Check sheet for the modelled part. Datum: model origin and axes. Units: mm. A direction names the side the tool comes from. Round coordinates to 2 decimals unless told otherwise and drop trailing zeros. Write each loop counter-clockwise with the first axis right and the second up, starting at its lowest first coordinate (ties: lowest second). Pieces come first, ordered by that corner, then holes. Notation, with made-up numbers: M 82.5,51 L 88.5,51 A16 ccw 88.5,73 Z; hole C -11.75,-38 d4. An arc over 180 degrees is marked long. Put each result on its own line as item: value.
Autodesk Inventor part; units mm, degrees
ref_plane "Work Plane1" through (0, 0, 0) normal (0, 0, 1) x (1, 0, 0)
ref_plane "Work Plane3" through (-57, -102.111, 0) normal (0, 1, 0) x (1, 0, 0)
ref_plane "YZ Plane" through (0, 0, 0) normal (1, 0, 0) x (0, 1, 0)
ref_plane "Work Plane1" through (0, 0, 0) normal (0, 0, 1) x (1, 0, 0)
sketch "Sketch1" plane through (0, 0, 0) normal (0, 0, 1) x (1, 0, 0)
  line L0 (-60, -142.911) -> (-60, -152.111) construction
  line L1 (0, -152.111) -> (-60, -152.111) construction
  line L2 (0, -142.911) -> (0, -152.111) construction
  line L3 (-57, -81.311) -> (-9.2, -81.311)
  line L4 (-9.2, -81.311) -> (-9.2, -142.911)
  line L5 (-9.2, -142.911) -> (-57, -142.911)
  line L6 (-57, -142.911) -> (-57, -81.311)
  line L7 (-57, -112.111) -> (-9.2, -112.111) construction
  line L8 (-57, -102.111) -> (-50, -102.111)
  line L9 (-50, -102.111) -> (-50, -122.111)
  line L10 (-50, -122.111) -> (-57, -122.111)
  line L11 (-57, -122.111) -> (-57, -102.111)
  line L12 (0, -142.911) -> (-60, -142.911)
  point P0 (0, 0)
  dimension "d0" = 20
  dimension "d1" = 7
extrude "Extrusion1" add sketch "Sketch1" against normal blind 1 contours L3 L4 L5 L6 L10 L9 L8
ref_plane "Work Plane2" through (-57, -112.111, 0) normal (0, 1, 0) x (1, 0, 0)
sketch "Sketch2" plane through (-57, -112.111, 0) normal (0, 1, 0) x (1, 0, 0)
  line L0 (7, 0) -> (0, 0) construction
  line L1 (7, 0) -> (7, 1) construction
  line L2 (0, 1) -> (7, 1) construction
  line L3 (0, 0) -> (0, 1) construction
  line L4 (0.0721, -0.8167) -> (0.0721, 1.0988)
  line L5 (0.0721, 1.0988) -> (-0.9279, 1.3644)
  line L6 (-0.9279, 1.3644) -> (0.0477, 5.0375)
  arc A0 (1.8249, 5.3661) -> (0.0477, 5.0375) centre (1.0142, 4.7807) ccw
  line L7 (1.8249, 5.3661) -> (4.3785, 1.8293)
  arc A1 (4.3785, 1.8293) -> (6, 1) centre (6, 3) ccw
  line L8 (6, 1) -> (7, 1)
  line L9 (7, 1) -> (7, 0)
  line L10 (7, 0) -> (6, 0)
  arc A2 (3.5677, 1.2439) -> (6, 0) centre (6, 3) ccw
  line L11 (3.5677, 1.2439) -> (1.0644, 4.7112)
  arc A3 (1.0644, 4.7112) -> (0.9749, 4.6822) centre (1.0243, 4.6822) ccw
  line L12 (47.8, 0) -> (0, 0)
  line L13 (47.8, 1) -> (0, 1)
  line L14 (6, 0) -> (6, 1) construction
  line L15 (0.9749, -0.9502) -> (0.9749, 4.6822)
  line L16 (0.2208, -1.01) -> (0.7236, -1.1435)
  arc A4 (0.7236, -1.1435) -> (0.9749, -0.9502) centre (0.7749, -0.9502) ccw
  arc A5 (0.0721, -0.8167) -> (0.2208, -1.01) centre (0.2721, -0.8167) ccw
  point P0 (57, 0)
  point P1 (0.9749, -1.2103)
  point P2 (0.0721, -0.9705)
  dimension "d8" = 1
  dimension "d9" = 1
  dimension "d11" = 1
  dimension "d12" = 0.0494
  dimension "d22" = 1
  dimension "d23" = 2
  dimension "d32" = 2
  dimension "d34" = 2.5
  dimension "d36" = 0.2
  dimension "d37" = 0.9874
  dimension "d38" = 1
  dimension "d39" = 125.829
  dimension "d40" = 3.8003
extrude "Extrusion2" add sketch "Sketch2" along normal mid plane 16 contours L4 L12 L15 A4 L16 A5 | L4 L13 L15 L12 | L4 L5 L6 A0 L7 A1 L13 A2 L11 A3 L15 | A2 L13 L8 L9 L10
ref_plane "Work Plane3" through (-57, -102.111, 0) normal (0, 1, 0) x (1, 0, 0)
sketch "Sketch4" plane through (-57, -102.111, 0) normal (0, 1, 0) x (1, 0, 0)
  line L0 (57, 0) -> (-3, 0) construction
  line L1 (0, 0) -> (47.8, 0) construction
  line L2 (47.8, 0) -> (47.8, 1) construction
  line L3 (0, 1) -> (47.8, 1) construction
  line L4 (0, 0) -> (0, 1) construction
  line L5 (0, 1) -> (47.8, 1)
  line L6 (45.8, 1) -> (47.8, 1)
  line L7 (47.8, 1) -> (49.8, 1)
  line L8 (49.8, 1) -> (49.8, 2.1)
  line L9 (49.4, 2.5) -> (46.2, 2.5)
  line L10 (45.8, 2.1) -> (45.8, 1)
  arc A0 (49.8, 2.1) -> (49.4, 2.5) centre (49.4, 2.1) ccw
  arc A1 (46.2, 2.5) -> (45.8, 2.1) centre (46.2, 2.1) ccw
  point P0 (49.8, 2.5)
  dimension "d25" = 1.5
  dimension "d26" = 2
  dimension "d27" = 2
  dimension "d28" = 0.4
extrude "Extrusion3" add sketch "Sketch4" along normal mid plane 4
mirror "Mirror1" about plane through (-57, -112.111, 0) normal (0, 1, 0) of "Extrusion3"
thicken "Thicken1" operation add thickness 0.1 both sides no extend neighbours yes toward (0, 1, 0) faces at (-25.1333, -142.911, -0.3333) (-57, -135.9777, -0.3333) (-9.2, -108.111, -0.3333) (-41.0667, -81.311, -0.3333) (-57, -95.1777, -0.3333)
equation "\"d8\" = d9"
properties part number "BAcA_3"
1. Cross-section at C-C (x = -42). Enter the section's corners in (y, z).
Computed values:
outline: M -142.81,-1 L -81.41,-1 L -81.41,0 L -142.81,0 Z
2. Cross-section at A-A (z = -4). Enter the section's corners in (x, y).
Computed values:
outline: M -57.23,-120.11 L -56.03,-120.11 L -56.03,-104.11 L -57.23,-104.11 Z; M -55.42,-120.11 L -54.19,-120.11 L -54.19,-104.11 L -55.42,-104.11 Z
3. Release check for a two-part mould opening along Y. For faces 5 (the flat face through (-9, -120.111, -2)), 6 (the flat face through (-54, -120.111, -3)), 7 (the flat face through (-54.7, -112.2, -3)), 8 (the flat face through (-9, -124.111, -2)) record: +Y half, -Y half, draft (parallel to the pull), parting line (faces both ways), or undercut.
Computed values:
face 5: undercut
face 6: undercut
face 7: draft
face 8: -Y half
4. Depth check by flat-ended pin: pin 1 Ø1.5 at (x, y) = (-35.5, -126) entering from +Z; pin 2 Ø1.6 at (x, y) = (-9.5, -123) entering from -Z; pin 3 Ø0.5 at (y, z) = (-137, -0.5) entering from -X. Enter the tip coordinate at first touch or a pass-through.
Computed values:
pin 1: stops at z = 0
pin 2: stops at z = -2.5
pin 3: stops at x = -56.9
5. Cross-section at D-D (y = -90). Enter the section's corners in (x, z).
Computed values:
outline: M -56.9,-1 L -9.3,-1 L -9.3,0 L -56.9,0 Z
6. Access from +Z, -Z, +X, -X, +Y, -Y to the whole of each face (thin tool, end or side, straight path). Record for faces 1 (the flat face through (-9, -100.111, -2)), 2 (the flat face through (-9, -104.111, -2)), 3 (the flat face through (-8, -122, -1)), 4 (the flat face through (-56.928, -112, 0)).
Computed values:
face 1: -Z, +X, -X, +Y
face 2: -Z, +X
face 3: +Z, +X, +Y, -Y
face 4: +Z, -X, +Y, -Y
7. Scan lines: probe 1 along Z at (x, y) = (-15.5, -93.5); probe 2 along X at (y, z) = (-114, -1.5); probe 3 along X at (y, z) = (-136, -0.75). Record each from-to range of solid material in increasing order.
Computed values:
probe 1: z = -1 to 0
probe 2: x = -57.89 to -56.03, -53.62 to -52.32
probe 3: x = -56.9 to -9.3
8. Cross-section at B-B (y = -105). Enter the section's corners in (x, z).
Computed values:
outline: M -57.93,-1.36 L -56.95,-5.04 A1 ccw -55.18,-5.37 L -52.62,-1.83 A2 cw -51,-1 L -9.3,-1 L -9.3,0 L -51,0 A3 ccw -53.43,-1.24 L -55.94,-4.71 A0.05 cw -56.03,-4.68 L -56.03,0.95 A0.2 ccw -56.28,1.14 L -56.78,1.01 A0.2 ccw -56.93,0.82 L -56.93,-1.1 Z
